Drawing for the job (mm, zero at the part's lowest x, y, z). Give positions to 0.01 mm unless a question says otherwise; leave off trailing zeros. Order: outer loops, then holes, each group sorted by start corner. A loop starts at its lowest first (then second) coordinate and runs counter-clockwise, first axis right, second up. Notation, with made-up numbers: (-14, 35) - (25, 35) arc R31 ccw to (25, 62) - close; hole circle Ø11 at (-19.5, 53). An arc over 180 degrees is marked (long way). Use a Markdown table: item, result.
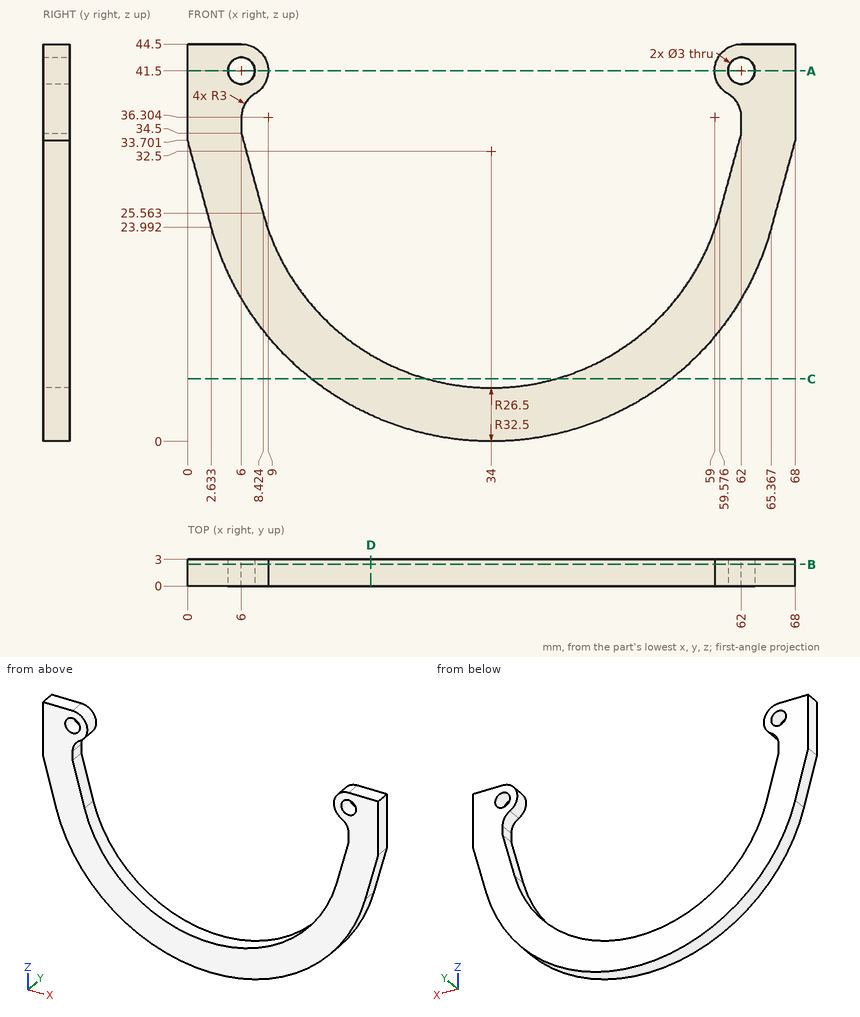
1) Slice it at C-C (z = 7). Write the cut outline in (x, y).
Computed:
| item | result |
|---|---|
| outline | (13.85, 0) - (26.79, 0) - (26.79, 3) - (13.85, 3) - close; (41.21, 0) - (54.15, 0) - (54.15, 3) - (41.21, 3) - close |
2) Pin check, flat tips, straight feed: P1, Ø3.5, axis at x = 62, z = 41.5, coming from the +Y side; P2, Ø1.5, axis at y = 2, z = 15, coming from the -X side. Stop position of each tip, or through.
Computed:
| item | result |
|---|---|
| P1 | stops at y = 3 |
| P2 | stops at x = 6.15 |
3) Wall check: line 1 (X direction, y = 2.05, z = 41.5); line 2 (X direction, y = 1.9, z = 40.5); line 3 (X direction, y = 2.55, z = 35.5). Give the ranges that are in metal, low to high. Write a range as from..to.
Computed:
| item | result |
|---|---|
| line 1 | x = 0..4.5, 7.5..9, 59..60.5, 63.5..68 |
| line 2 | x = 0..4.88, 7.12..8.83, 59.17..60.88, 63.12..68 |
| line 3 | x = 0..6, 62..68 |
4) Slice it at D-D (x = 20.5). Write the cut outline in (y, z), and give its area (3 significant figures).
Computed:
| item | result |
|---|---|
| outline | (0, 2.94) - (3, 2.94) - (3, 9.7) - (0, 9.7) - close |
| area | 20.3 mm² |
5) Slice it at A-A (z = 41.5). Write the cut outline in (x, y).
Computed:
| item | result |
|---|---|
| outline | (0, 0) - (4.5, 0) - (4.5, 3) - (0, 3) - close; (7.5, 0) - (9, 0) - (9, 3) - (7.5, 3) - close; (59, 0) - (60.5, 0) - (60.5, 3) - (59, 3) - close; (63.5, 0) - (68, 0) - (68, 3) - (63.5, 3) - close |
6) Slice it at B-B (y = 2.45). Write the cut outline in (x, z).
Computed:
| item | result |
|---|---|
| outline | (0, 33.7) - (2.63, 23.99) arc R32.5 ccw to (65.37, 23.99) - (68, 33.7) - (68, 44.5) - (62, 44.5) arc R3 ccw to (60.5, 38.9) arc R3 cw to (62, 36.3) - (62, 34.5) - (59.58, 25.56) arc R26.5 cw to (8.42, 25.56) - (6, 34.5) - (6, 36.3) arc R3 cw to (7.5, 38.9) arc R3 ccw to (6, 44.5) - (0, 44.5) - close; hole circle Ø3 at (6, 41.5); hole circle Ø3 at (62, 41.5) |
